The figure shows three views and two pictorial views of one solid part (mm, origin at its lowest corner). Answer the questions. A direction names the side the tool comes from. Round coordinates to 2 decimals unless told otherwise and drop trailing zeros. Write each loop counter-clockwise with the first axis right and the second up, starting at its lowest first coordinate (ties: lowest second). Pieces come first, ordered by that corner, then holes. Notation, with made-up numbers: (-15.5, -17.5) -> (-6.5, -17.5) arc R14 cw to (-6.5, -2.5) -> close; hole circle Ø4 at (-13, 29.25). An arc over 180 degrees is marked (long way). One line per item, written item: value.
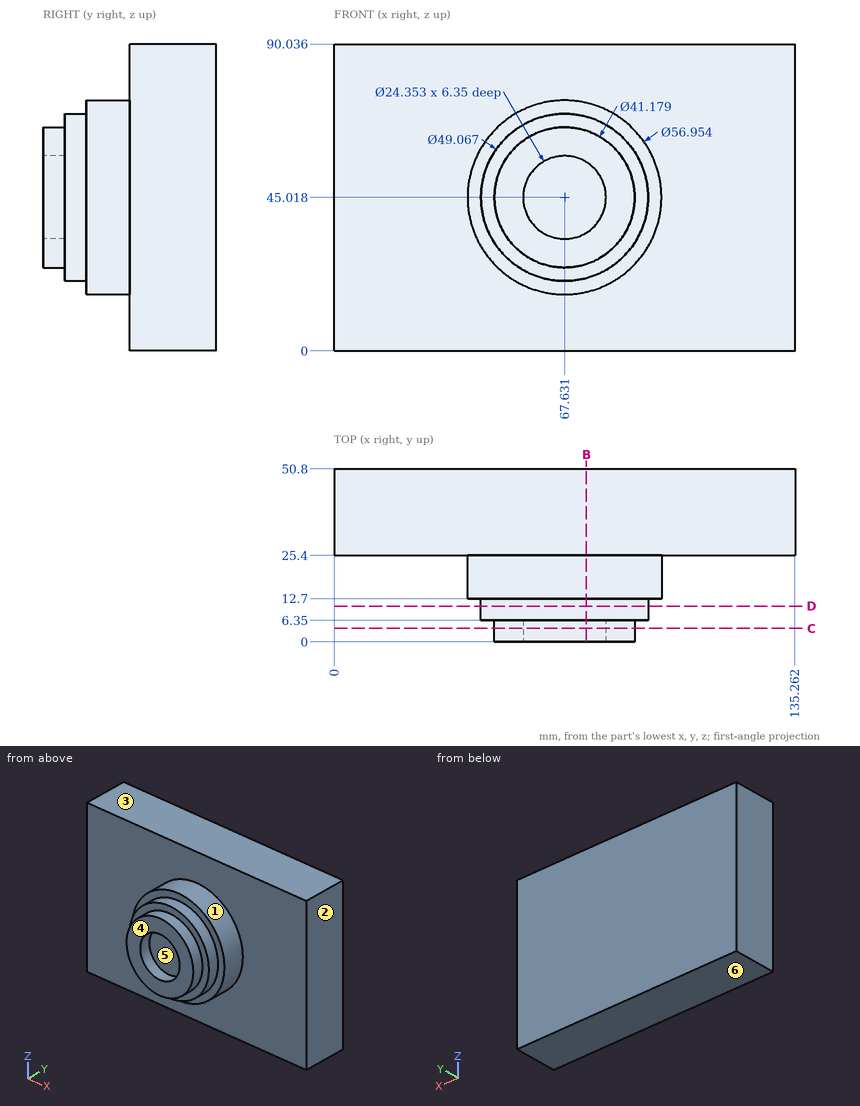
(1) Find section C-C on y = 4. Give the vertices of the cut face in (x, z), plus the area to 3 significant figures.
Reported:
outline: circle Ø41.18 at (67.63, 45.02); hole circle Ø24.35 at (67.63, 45.02)
area: 866 mm2
(2) A tool of negligible diameter and unlimited length cuts with its end or side. For the marked faces 1 and 2, from which of +Z, -Z, +X, -X, +Y, -Y can it reach the whole face along a straight path? Write none if from no direction.
Reported:
face 1: -Y
face 2: +Z, -Z, +X, +Y, -Y
(3) Find section B-B on x = 74. Give the vertices of the cut face in (y, z), plus the area to 3 significant figures.
Reported:
outline: (0, 25.44) -> (6.35, 25.44) -> (6.35, 21.33) -> (12.7, 21.33) -> (12.7, 17.26) -> (25.4, 17.26) -> (25.4, 0) -> (50.8, 0) -> (50.8, 90.04) -> (25.4, 90.04) -> (25.4, 72.77) -> (12.7, 72.77) -> (12.7, 68.71) -> (6.35, 68.71) -> (6.35, 64.6) -> (0, 64.6) -> (0, 55.4) -> (6.35, 55.4) -> (6.35, 34.64) -> (0, 34.64) -> close
area: 3,410 mm2
(4) Flat-ended cylindrical pins translate along their axes: pin 1 Ø4 at (x, z) = (110.5, 19) entering from -Y; pin 2 Ø8 at (y, z) = (14, 33) entering from +X (1 decimal); pin 3 Ø14.5 at (x, z) = (67.63, 45.02) entering from -Y. Find the tip coordinate at first contact, or state that the pin passes through.
Reported:
pin 1: stops at y = 25.4
pin 2: stops at x = 95
pin 3: stops at y = 6.35
(5) Consider probe 1 along Y at (x, z) = (16, 17); probe 2 along X at (y, z) = (8, 39) (1 decimal); probe 3 along Y at (x, z) = (58, 66). Determine where each line is inside the solid, lowest interval first.
Reported:
probe 1: y = 25.4 to 50.8
probe 2: x = 43.8 to 91.4
probe 3: y = 6.35 to 50.8
(6) For a pull along Z with two mould halves and no side action, classify the marked faces 3, 4, 5 and 6 as pulls with the +Z half, pulls with the -Z half, needs draft (parallel to the pull), parting line crosses it, or undercut.
Reported:
face 3: pulls with the +Z half
face 4: needs draft
face 5: undercut
face 6: pulls with the -Z half
(7) Find section D-D on y = 10.5. Give the vertices of the cut face in (x, z) (1 decimal).
Reported:
outline: circle Ø49.1 at (67.6, 45)
